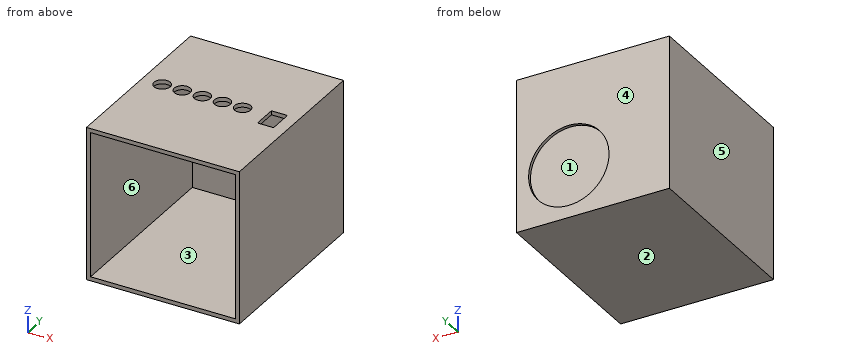
from build123d import *

# Parameters (mm, degrees)
SKETCH2_W           = 90
SKETCH2_H           = 90
BOSS_EXTRUDE2_DEPTH = 110
SHELL2_T            = 2.5
SKETCH3_R           = 5
SKETCH3_W           = 10
SKETCH3_H           = 15
CUT_EXTRUDE1_DEPTH  = 10
SKETCH4_R           = 25
CUT_EXTRUDE2_DEPTH  = 2


with BuildPart() as part:
    # Sketch2 → Boss-Extrude2 (new body)
    with BuildSketch(Plane(origin=(0, 0, 0), x_dir=(1, 0, 0), z_dir=(0, 1, 0))):
        Rectangle(SKETCH2_W, SKETCH2_H)
    extrude(amount=BOSS_EXTRUDE2_DEPTH)

    # Shell2
    shell2_openings = [part.faces().sort_by_distance(p)[0] for p in [
        (0, 0, 0),
    ]]
    offset(amount=SHELL2_T, openings=shell2_openings, kind=Kind.INTERSECTION)

    # Sketch3 → Cut-Extrude1 (cut)
    with BuildSketch(Plane.XY.offset(47.5)):
        with Locations((-35, 60)):
            Circle(SKETCH3_R)
        with Locations((-22.5, 60)):
            Circle(SKETCH3_R)
        with Locations((-10, 60)):
            Circle(SKETCH3_R)
        with Locations((2.5, 60)):
            Circle(SKETCH3_R)
        with Locations((15, 60)):
            Circle(SKETCH3_R)
        with Locations((35, 57.5)):
            Rectangle(SKETCH3_W, SKETCH3_H)
    extrude(amount=-CUT_EXTRUDE1_DEPTH, mode=Mode.SUBTRACT)

    # Sketch4 → Cut-Extrude2 (cut)
    with BuildSketch(Plane(origin=(0, 112.5, 0), x_dir=(1, 0, 0), z_dir=(0, 1, 0))):
        with Locations(Location((15, 15, 0), (0, 0, 270))):
            Circle(SKETCH4_R)
    extrude(amount=-CUT_EXTRUDE2_DEPTH, mode=Mode.SUBTRACT)


solid = part.part
CAD build for the part. Positions are in the model's coordinates, mm. Face numbers are marked on the shaded views. A direction names the side the tool comes from. Coordinates: 2 decimals unless noted, no trailing zeros. Loops run counter-clockwise (first coordinate to the right, second up) from the corner with the lowest first, then second, coordinate; pieces in that order, holes last. Notation, with made-up numbers: (-3, 60.5) - (30, 60.5) arc R25 ccw to (30, 80.5) - close; hole circle Ø7 at (37, 12). An arc over 180 degrees is marked (long way). Use one line per item in the form item = value. Start each with the question number.
1) Flat gauge pin, fed straight in: pin 1 (10 mm diameter, centred on x = 11.5, z = 17, fed in from -Y). Where does the tip first touch, or does it go through?
2) Two-plate mould, pull along Z, no slides. Class the marked faces 1, 2, 3 and 4: +Z half, -Z half, draft (parallel to the pull), parting line (faces both ways), or undercut.
3) Band-saw the part on C-C (z = 5). Give the cut face in (x, y), and give its area (4 significant figures).
4) Band-saw the part on D-D (x = -35). Give the cut face in (y, z), and give its area (4 significant figures).
5) Tool access for the marked faces 5 and 6: list every direction of +Z, -Z, +X, -X, +Y, -Y with a clear straight run to the whole face (end or side of a thin tool).
6) Drill centre lines: L1, parallel to X at y = 10, z = -20.5; L2, parallel to Y at x = -10, z = 46.6. Where is each one in solid material? Low to high. Write a range as from..to.
7) Band-saw the part on B-B (x = 15). Give the cut face in (y, z), and give its area (4 significant figures).
8) Band-saw the part on A-A (y = 18). Give the cut face in (x, z), and give its area (3 significant figures).
Check values:
q1.pin_1 = 110
q2.face_1 = undercut
q2.face_2 = -Z half
q2.face_3 = undercut
q2.face_4 = draft
q3.outline = (-47.5, 0) - (-45, 0) - (-45, 110) - (45, 110) - (45, 0) - (47.5, 0) - (47.5, 112.5) - (30, 112.5) - (30, 110.5) - (0, 110.5) - (0, 112.5) - (-47.5, 112.5) - close
q3.area = 727.5 mm2
q4.outline = (0, -47.5) - (112.5, -47.5) - (112.5, 47.5) - (65, 47.5) - (65, 45) - (110, 45) - (110, -45) - (0, -45) - close; (0, 45) - (55, 45) - (55, 47.5) - (0, 47.5) - close
q4.area = 762.5 mm2
q5.face_5 = +Z, -Z, -X, +Y, -Y
q5.face_6 = -Y
q6.L1 = -47.5..-45, 45..47.5
q6.L2 = 0..55, 65..112.5
q7.outline = (0, -47.5) - (112.5, -47.5) - (112.5, -40) - (110.5, -40) - (110.5, 10) - (112.5, 10) - (112.5, 47.5) - (65, 47.5) - (65, 45) - (110, 45) - (110, -45) - (0, -45) - close; (0, 45) - (55, 45) - (55, 47.5) - (0, 47.5) - close
q7.area = 662.5 mm2
q8.outline = (-47.5, -47.5) - (47.5, -47.5) - (47.5, 47.5) - (-47.5, 47.5) - close; hole (-45, -45) - (45, -45) - (45, 45) - (-45, 45) - close
q8.area = 925 mm2
